Build history of the part. All positions in model axes, mm. A direction names the side the tool comes from. Round coordinates to 2 decimals unless told otherwise and drop trailing zeros. Loops run counter-clockwise (first coordinate to the right, second up) from the corner with the lowest first, then second, coordinate; pieces in that order, holes last. Notation, with made-up numbers: (-14.75, 82.25) - (34.25, 82.25) arc R15 ccw to (34.25, 110.25) - close; hole circle Ø4 at (81.5, 78.25). An arc over 180 degrees is marked (long way). Put each result on its own line as item: value. Start each with the question number.
from build123d import *

# Parameters (mm, degrees)
BOSS_EXTRUDE2_DEPTH = 80
BOSS_EXTRUDE3_DEPTH = 10
SKETCH1_9_W         = 15
SKETCH1_9_H         = 8
BOSS_EXTRUDE4_DEPTH = 40
CUT_EXTRUDE1_DEPTH  = 108.721864076
SKETCH3_W           = 18
SKETCH3_H           = 43
CUT_EXTRUDE2_DEPTH  = 133.759180474


with BuildPart() as part:
    # Sketch1 → Boss-Extrude2 (new body)
    with BuildSketch(Plane(origin=(0, 0, 0), x_dir=(1, 0, 0), z_dir=(0, 1, 0))):
        with BuildLine():
            Line((11, 17), (11, 22.449944321))
            ThreePointArc((11, 22.449944321), (0, 25), (-11, 22.449944321))
            Line((-11, 22.449944321), (-11, 17))
            Line((-11, 17), (-11, 9))
            Line((-11, 9), (-11, -9))
            Line((-11, -9), (-11, -17))
            Line((-11, -17), (-11, -22.449944321))
            ThreePointArc((-11, -22.449944321), (0, -25), (11, -22.449944321))
            Line((11, -22.449944321), (11, -17))
            Line((11, -17), (11, -9))
            Line((11, -9), (11, 9))
            Line((11, 9), (11, 17))
        make_face()
    extrude(amount=BOSS_EXTRUDE2_DEPTH)

    # Sketch1_6 → Boss-Extrude3 (add)
    with BuildSketch(Plane(origin=(0, 0, 0), x_dir=(1, 0, 0), z_dir=(0, 1, 0))):
        with BuildLine():
            ThreePointArc((-11, 22.449944321), (0, 25), (11, 22.449944321))
            ThreePointArc((11, 22.449944321), (14.916170372, 20.062598571), (18.33030278, 17))
            Line((18.33030278, 17), (30.594117082, 17))
            ThreePointArc((30.594117082, 17), (0, 35), (-30.594117082, 17))
            Line((-30.594117082, 17), (-18.33030278, 17))
            ThreePointArc((-18.33030278, 17), (-14.916170372, 20.062598571), (-11, 22.449944321))
        make_face()
        with BuildLine():
            ThreePointArc((18.33030278, -17), (14.916170372, -20.062598571), (11, -22.449944321))
            ThreePointArc((11, -22.449944321), (0, -25), (-11, -22.449944321))
            ThreePointArc((-11, -22.449944321), (-14.916170372, -20.062598571), (-18.33030278, -17))
            Line((-18.33030278, -17), (-30.594117082, -17))
            ThreePointArc((-30.594117082, -17), (0, -35), (30.594117082, -17))
            Line((30.594117082, -17), (18.33030278, -17))
        make_face()
    extrude(amount=BOSS_EXTRUDE3_DEPTH)

    # Sketch1_9 → Boss-Extrude4 (add)
    with BuildSketch(Plane(origin=(0, 0, 0), x_dir=(1, 0, 0), z_dir=(0, 1, 0))):
        with Locations((-42.5, 13)):
            Rectangle(SKETCH1_9_W, SKETCH1_9_H)
        Polygon((-11, 9), (-11, 17), (-18.33030278, 17), (-30.594117082, 17), (-35, 17), (-35, 9), align=None)
        Polygon((-11, -9), (-11, 9), (-35, 9), (-50, 9), (-50, -9), (-35, -9), align=None)
        with Locations((-42.5, -13)):
            Rectangle(SKETCH1_9_W, SKETCH1_9_H)
        Polygon((-11, -17), (-11, -9), (-35, -9), (-35, -17), (-30.594117082, -17), (-18.33030278, -17), align=None)
        with Locations((42.5, -13)):
            Rectangle(SKETCH1_9_W, SKETCH1_9_H)
        Polygon((35, -9), (11, -9), (11, -17), (18.33030278, -17), (30.594117082, -17), (35, -17), align=None)
        Polygon((35, 9), (11, 9), (11, -9), (35, -9), (50, -9), (50, 9), align=None)
        Polygon((18.33030278, 17), (11, 17), (11, 9), (35, 9), (35, 17), (30.594117082, 17), align=None)
        with Locations((42.5, 13)):
            Rectangle(SKETCH1_9_W, SKETCH1_9_H)
        with BuildLine():
            ThreePointArc((18.33030278, 17), (14.916170372, 20.062598571), (11, 22.449944321))
            Line((11, 22.449944321), (11, 17))
            Line((11, 17), (18.33030278, 17))
        make_face()
        with BuildLine():
            Line((-11, 17), (-11, 22.449944321))
            ThreePointArc((-11, 22.449944321), (-14.916170372, 20.062598571), (-18.33030278, 17))
            Line((-18.33030278, 17), (-11, 17))
        make_face()
        with BuildLine():
            Line((-11, -22.449944321), (-11, -17))
            Line((-11, -17), (-18.33030278, -17))
            ThreePointArc((-18.33030278, -17), (-14.916170372, -20.062598571), (-11, -22.449944321))
        make_face()
        with BuildLine():
            Line((18.33030278, -17), (11, -17))
            Line((11, -17), (11, -22.449944321))
            ThreePointArc((11, -22.449944321), (14.916170372, -20.062598571), (18.33030278, -17))
        make_face()
    extrude(amount=BOSS_EXTRUDE4_DEPTH)

    # Sketch2 → Cut-Extrude1 (cut, through all)
    with BuildSketch(Plane.XY.offset(17)):
        Polygon((-50, 10), (-35, 40), (-50, 40), align=None)
        Polygon((50, 10), (35, 40), (50, 40), align=None)
    extrude(amount=-CUT_EXTRUDE1_DEPTH, mode=Mode.SUBTRACT)

    # Sketch3 → Cut-Extrude2 (cut, through all)
    with BuildSketch(Plane.ZY.offset(50)):
        with Locations((0, 41.5)):
            Rectangle(SKETCH3_W, SKETCH3_H)
    extrude(amount=-CUT_EXTRUDE2_DEPTH, mode=Mode.SUBTRACT)


solid = part.part
Item 1: Which spindle directions (+Z, -Z, +X, -X, +Y, -Y) get a long thin tool onto all of the face, cutting with end or side? Do faces 1 (the flat face through (-34, 20, -17)), 2 (the flat face through (-11, 64, 0)), 3 (the flat face through (-1, 20, 0)). Say none if no direction does.
Item 2: Two-plate mould, pull along Z, no slides. Class faces 4 (the flat face through (34, 20, 17)), 5 (the flat face through (0, 63, 0)), 6 (the flat face through (-1, 36, -9)), 7 (the flat face through (-23, 40, 14)): pulls with the +Z half, pulls with the -Z half, needs draft (parallel to the pull), parting line crosses it, or undercut.
Item 3: Drill centre lines: probe 1 along Z at (x, y) = (24.5, 35.5); probe 2 along X at (y, z) = (43, -16); probe 3 along Y at (x, z) = (6, 26.5). Where is each one in solid material? Low to high. Write a range as [from, to].
Item 4: Slice it at D-D (y = 14.5). Give the cut face in (x, z), plus the area to 3 significant figures.
Item 5: Slice it at C-C (x = -42.5). Give the cut face in (y, z), plus the area to 3 significant figures.
Item 6: Drop flat-ended pins along their axis: pin 1 Ø15 at (x, z) = (21, -16.5) entering from +Y; pin 2 Ø9.5 at (x, y) = (-35, 10.5) entering from +Z; pin 3 Ø13 at (x, y) = (-15, 32.5) entering from -Z. Give the stop position or say it passes through.
Item 7: Slice it at A-A (z = 0.5). Give the cut face in (x, y).
Item 8: Slice it at B-B (y = 28.5). Give the cut face in (x, z).
Computed values:
1. face 1: -Z, -X, +Y
1. face 2: +Z, -Z, -X, +Y
1. face 3: +X, -X
2. face 4: pulls with the +Z half
2. face 5: undercut
2. face 6: undercut
2. face 7: needs draft
3. probe 1: z = [-17, -9], [9, 17]
3. probe 2: x = [-11, 11]
3. probe 3: y = [0, 10]
4. outline: (-47.75, -17) - (-18.33, -17) arc R25 ccw to (18.33, -17) - (47.75, -17) - (47.75, 17) - (18.33, 17) arc R25 ccw to (-18.33, 17) - (-47.75, 17) - close
4. area: 3,650 mm^2
5. outline: (0, -17) - (25, -17) - (25, -9) - (20, -9) - (20, 9) - (25, 9) - (25, 17) - (0, 17) - close
5. area: 760 mm^2
6. pin 1: stops at y = 40
6. pin 2: stops at z = 17.56
6. pin 3: stops at z = -23.51
7. outline: (-50, 0) - (50, 0) - (50, 10) - (45, 20) - (-45, 20) - (-50, 10) - close; (-11, 63) - (11, 63) - (11, 80) - (-11, 80) - close
8. outline: (-40.75, -17) - (-18.33, -17) arc R25 ccw to (18.33, -17) - (40.75, -17) - (40.75, -9) - (-40.75, -9) - close; (-40.75, 9) - (40.75, 9) - (40.75, 17) - (18.33, 17) arc R25 ccw to (-18.33, 17) - (-40.75, 17) - close
